Verification items for the finished model (mm, model axes). Face numbers are marked on the shaded views. Give positions to 0.01 mm unless a question says otherwise; leave off trailing zeros. Order: outer loops, then holes, each group sorted by start corner. A loop starts at its lowest first (then second) coordinate and runs counter-clockwise, first axis right, second up. Notation, with made-up numbers: M 69,61 L 99,61 A14 cw 99,80 Z; hole C 25.25,-3 d7. An arc over 180 degrees is marked long. Answer as a JSON object with one key per item and string values.
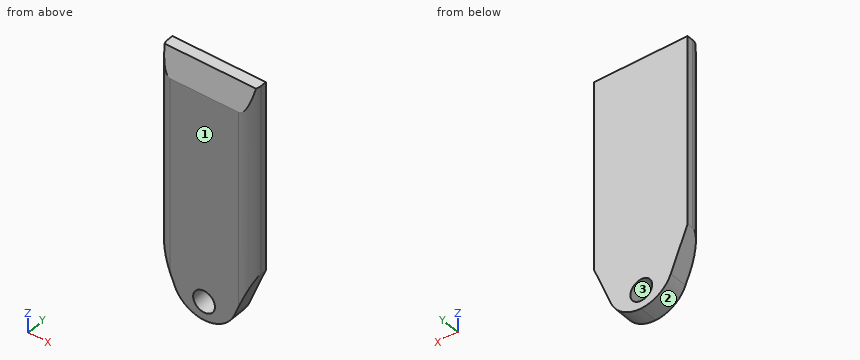
```python
from build123d import *

# Parameters (mm, degrees)
CROQUIS1_W              = 15
CROQUIS1_H              = 3
SALIENTE_EXTRUIR1_DEPTH = 40.5
CROQUIS2_OUTSIDE_W      = 25.658
CROQUIS2_OUTSIDE_H      = 51.158
CROQUIS2_OUTSIDE_W_2    = 15
CROQUIS2_OUTSIDE_H_2    = 40.5
CROQUIS2_OUTSIDE_R      = 1.75
CORTAR_EXTRUIR1_DEPTH   = 40.5
CHAFL_N1_SIZE           = 4
CHAFL_N1_SIZE2          = 1.2
CHAFL_N2_SIZE           = 4
CHAFL_N2_SIZE2          = 10
REDONDEO1_R             = 2
REDONDEO2_R             = 5.169615


with BuildPart() as part:
    # Croquis1 → Saliente-Extruir1 (new body)
    with BuildSketch(Plane.XY):
        with Locations((0, 108.5)):
            Rectangle(CROQUIS1_W, CROQUIS1_H)
    extrude(amount=-SALIENTE_EXTRUIR1_DEPTH)

    # Croquis2 outside → Cortar-Extruir1 (cut)
    # profile 1 of 2: a face of its own
    with BuildSketch(Plane.XZ.offset(-107)):
        with Locations((0, -20.25)):
            Rectangle(CROQUIS2_OUTSIDE_W, CROQUIS2_OUTSIDE_H)
        with Locations((0, -20.25)):
            Rectangle(CROQUIS2_OUTSIDE_W_2, CROQUIS2_OUTSIDE_H_2, mode=Mode.SUBTRACT)
    # profile 2 of 2: a face of its own
    with BuildSketch(Plane.XZ.offset(-107)):
        with Locations(Location((-0.065549886, -37.5, 0), (0, 0, 270))):
            Circle(CROQUIS2_OUTSIDE_R)
    extrude(amount=-CORTAR_EXTRUIR1_DEPTH, mode=Mode.SUBTRACT)

    # Chaflán1
    chafl_n1_edges = [part.edges().sort_by_distance(p)[0] for p in [
        (0, 107, 0),
    ]]
    chafl_n1_side = [part.faces().sort_by_distance(p)[0] for p in [
        (0.001054835, 107, -19.972411249),
    ]]
    chamfer(chafl_n1_edges, length=CHAFL_N1_SIZE, length2=CHAFL_N1_SIZE2, reference=chafl_n1_side[0])

    # Chaflán2
    chafl_n2_edges = [part.edges().sort_by_distance(p)[0] for p in [
        (7.5, 108.5, -40.5),
        (-7.5, 108.5, -40.5),
    ]]
    chafl_n2_side = [part.faces().sort_by_distance(p)[0] for p in [
        (0, 108.5, -40.5),
    ]]
    chamfer(chafl_n2_edges, length=CHAFL_N2_SIZE, length2=CHAFL_N2_SIZE2, reference=chafl_n2_side[0])

    # Redondeo1
    redondeo1_edges = [part.edges().sort_by_distance(p)[0] for p in [
        (-7.5, 107, -17.25),
        (7.5, 107, -17.25),
    ]]
    fillet(redondeo1_edges, radius=REDONDEO1_R)

    # Redondeo2
    redondeo2_edges = [part.edges().sort_by_distance(p)[0] for p in [
        (3.5, 108.5, -40.5),
        (-3.5, 108.5, -40.5),
    ]]
    fillet(redondeo2_edges, radius=REDONDEO2_R)


solid = part.part
```
Q1. Release check for a two-part mould opening along Z. For the marked faces 1, 2 and 3 record: +Z half, -Z half, draft (parallel to the pull), parting line (faces both ways), or undercut.
Resolved:
{"face 1": "draft", "face 2": "-Z half", "face 3": "undercut"}
Q2. Section check D-D on y = 109.55. Record the cut outline in (x, z).
Resolved:
{"outline": "M -7.5,-30.5 L -4.8,-37.25 A5.17 ccw 4.8,-37.25 L 7.5,-30.5 L 7.5,0 L -7.5,0 Z; hole C -0.07,-37.5 d3.5"}
Q3. Section check C-C on y = 107.45. Record the cut outline in (x, z), then the cut area to 3 significant figures.
Resolved:
{"outline": "M -6.76,-32.34 L -4.8,-37.25 A5.17 ccw 4.8,-37.25 L 6.76,-32.34 L 6.76,-2.5 L -6.76,-2.5 Z; hole C -0.07,-37.5 d3.5", "area": "473 mm²"}
Q4. Material ranges on L1, parallel to X at y = 108.1, z = -37.5; L2, parallel to Z at x = -0.25, y = 108.55; L3, parallel to X at y = 108.05, z = -18.5, recorded low to high.
Resolved:
{"L1": "x = -4.69 to -1.82, 1.68 to 4.69", "L2": "z = -40.49 to -39.24, -35.76 to 0", "L3": "x = -7.26 to 7.26"}
Q5. Section check B-B on z = -14. Record the cut outline in (x, y).
Resolved:
{"outline": "M -7.5,109 A2 ccw -5.5,107 L 5.5,107 A2 ccw 7.5,109 L 7.5,110 L -7.5,110 Z"}
Q6. Section check A-A on x = -1. Record the cut outline in (y, z).
Resolved:
{"outline": "M 107,-40.4 L 110,-40.4 L 110,-38.98 L 107,-38.98 Z; M 107,-36.02 L 110,-36.02 L 110,0 L 108.2,0 L 107,-4 Z"}
Q7. Gauge pin test, flat ends, axial feed: pin 1 Ø1.5 at (y, z) = (107.5, -12) entering from -X; pin 2 Ø3 at (x, z) = (-0.07, -37.5) entering from -Y; pin 3 Ø1 at (y, z) = (107.5, -20.5) entering from +X. Record the tip position at first contact, or that the pin passes through.
Resolved:
{"pin 1": "stops at x = -7.35", "pin 2": "passes through", "pin 3": "stops at x = 7.23"}
